Model file for the job. Use its own axes, mm. A direction names the side the tool comes from. Round coordinates to 2 decimals unless told otherwise and drop trailing zeros. Order: outer loops, then holes, each group sorted by start corner. A loop starts at its lowest first (then second) coordinate and runs counter-clockwise, first axis right, second up. Notation, with made-up numbers: (-16, 12.25) - (-3, 12.25) arc R10 ccw to (-3, 30.25) - close; hole circle Ø3 at (-27.5, -6.75). An arc over 180 degrees is marked (long way). Answer as CSV lines item,"result". Start each with the question number.
1. Wall check: line 1 along X through (y, z) = (0.65, -45.5). Give the ranges that are in metal, low to high. Write a range as [from, to].
2. 3-axis set-ups, long thin cutter, end or side, ignore diameter. For faces 4 (the face through (-56, 0.394, -46.454)), 5 (the face through (3, 17, 7.393)), 6 (the face through (-3.9, 7.5, 8.5)), 7 (the face through (5.4, 13, 8)), 8 (the face through (-63.1, 7.9, -45.5)): which of +Z, -Z, +X, -X, +Y, -Y reach the whole face in a straight line?
3. Band-saw the part on D-D on x = -22.5. List the corners of the cut face in (y, z), then the cut area to 3 significant figures.
4. Band-saw the part on A-A on x = 2.7. State how many separate pieces and enclosed holes the cut face has, then the cut area to 3 significant figures.
5. Band-saw the part on B-B on y = 20.5. List the corners of the cut face in (x, z).
6. Band-saw the part on C-C on z = 3.5. List the corners of the cut face in (x, y).
7. Pull direction Z, two halves, no side cores. Call faces 1 (the face through (-3.9, 7.5, -50.4)), 2 (the face through (-63, 3.8, -21)), 3 (the face through (-27, 3, -51)): released by +Z, released by -Z, zero draft, split by the parting line, or undercut.
8. Pin check, flat tips, straight feed: pin 1 Ø1.3 at (x, z) = (-24.5, -50.5) entering from +Y; pin 2 Ø1.6 at (x, z) = (-55.7, 3.5) entering from +Y. Stop position of each tip, or through.
```python
from build123d import *

# Parameters (mm, degrees)
SKETCH1_R            = 0.9999999999999983
SKETCH1_R_2          = 1.0000000000000002
SKETCH1_R_3          = 1.0000000000000013
BOSS_EXTRUDE1_DEPTH  = 0.8
BOSS_EXTRUDE2_DEPTH  = 3
SKETCH3_W            = 2.6000000000000014
SKETCH3_H            = 1.6000000000000156
SKETCH3_W_2          = 5.400000000000002
SKETCH3_H_2          = 1.6066889909461715
SKETCH3_H_3          = 1.6000000000000094
BOSS_EXTRUDE3_DEPTH  = 27
LOFT4_START          = 7.4
LOFT4_DEPTH          = 1.6
LOFT4_START_2        = 7.403174683
LOFT4_2_DEPTH        = 0.596825317
MIRROR6_START        = 7.4
MIRROR6_COPY_1_DEPTH = 1.6
MIRROR6_START_2      = 7.403174683
MIRROR6_COPY_2_DEPTH = 0.596825317
MIRROR6_COPY_3_DEPTH = 1.6
MIRROR6_COPY_4_DEPTH = 0.596825317


with BuildPart() as part:
    # Sketch1 → Boss-Extrude1 (new body)
    with BuildSketch(Plane(origin=(0, 0, 0), x_dir=(1, 0, 0), z_dir=(0, 1, 0))):
        Polygon((0, 0), (5.4, 0), (5.400000000000007, -7.000000000000003), (5.400000000000002, -8.999999999999995), (-58.4, -8.999999999999995), (-61.40000000000001, -8.999999999999995), (-64.4, -8.999999999999995), (-64.4, 51), (-61.40000000000001, 51), (-58.4, 51), (5.400000000000004, 50.99999999999999), (5.400000000000004, 48.99999999999999), (5.4, 42.00000000000001), (0, 41.99999999999999), (-6.07e-15, 48.99999999999999), (-53.00000000000001, 48.99999999999999), (-53.00000000000001, 41.99999999999999), (-58.400000000000006, 41.99999999999999), (-61.40000000000001, 41.99999999999999), (-61.40000000000001, 0), (-58.400000000000006, 0), (-53.00000000000001, -1.73e-15), (-53.00000000000001, -6.999999999999986), (-6.14e-15, -6.999999999999999), align=None)
        with Locations(Location((-55.70000000000001, -3.4999999999999885, 0), (0, 0, 270))):
            Circle(SKETCH1_R, mode=Mode.SUBTRACT)
        with Locations(Location((2.700000000000006, -3.499999999999999, 0), (0, 0, 270))):
            Circle(SKETCH1_R_2, mode=Mode.SUBTRACT)
        with Locations(Location((2.7000000000000015, 45.5, 0), (0, 0, 90))):
            Circle(SKETCH1_R_3, mode=Mode.SUBTRACT)
        with Locations(Location((-55.7, 45.5, 0), (0, 0, 90))):
            Circle(SKETCH1_R, mode=Mode.SUBTRACT)
    extrude(amount=BOSS_EXTRUDE1_DEPTH)

    # Sketch2 → Boss-Extrude2 (add)
    with BuildSketch(Plane(origin=(0, 0.8, 0), x_dir=(1, 0, 0), z_dir=(0, 1, 0))):
        Polygon((-64.4, 51), (5.400000000000002, 51), (5.400000000000002, 49.39999999999999), (-61.800000000000004, 49.39999999999999), (-61.800000000000004, -7.399999999999985), (5.400000000000009, -7.399999999999985), (5.400000000000002, -8.999999999999995), (-64.4, -8.999999999999995), align=None)
    extrude(amount=BOSS_EXTRUDE2_DEPTH)

    # Sketch3 → Boss-Extrude3 (add)
    with BuildSketch(Plane(origin=(0, 3.8, 0), x_dir=(1, 0, 0), z_dir=(0, 1, 0))):
        with Locations((-63.10000000000001, 50.2)):
            Rectangle(SKETCH3_W, SKETCH3_H)
        with Locations((2.700000000000001, 50.2)):
            Rectangle(SKETCH3_W_2, SKETCH3_H)
        with Locations((2.700000000000001, -8.196655504526909)):
            Rectangle(SKETCH3_W_2, SKETCH3_H_2)
        with Locations((-63.10000000000001, -8.19999999999999)):
            Rectangle(SKETCH3_W, SKETCH3_H_3)
    extrude(amount=BOSS_EXTRUDE3_DEPTH)

    # Sketch9 → Loft3 section 0
    with BuildSketch(Plane(origin=(0, 3.8, 0), x_dir=(1, 0, 0), z_dir=(0, 1, 0))):
        with BuildLine():
            Line((-64.4, -7.399999999999985), (-64.4, 0.6000000000000146))
            Line((-64.4, 0.6000000000000146), (-61.800000000000004, 0.6000000000000149))
            Line((-61.800000000000004, 0.6000000000000149), (-61.800000000000004, -7.399999999999985))
            Line((-61.800000000000004, -7.399999999999985), (-64.4, -7.399999999999985))
        make_face()
    # Sketch7 → Loft3 section 1
    with BuildSketch(Plane(origin=(0, 0, 7.399999999999985), x_dir=(-1, 0, -3.903e-14), z_dir=(3.903e-14, 0, -1))):
        with BuildLine():
            Line((64.40000000000235, 3.8), (64.4000000000023, 11.799999999999999))
            Line((64.4000000000023, 11.799999999999999), (61.80000000000229, 11.799999999999997))
            Line((61.80000000000229, 11.799999999999997), (61.80000000000229, 3.8))
            Line((61.80000000000229, 3.8), (64.40000000000235, 3.8))
        make_face()
    loft3 = loft()

    # Loft4: read off the stored shape, not the designer's step
    # Loft4 outline → Loft4 (add)
    with BuildSketch(Plane.XY.offset(LOFT4_START)):
        Polygon((-61.8, 11.8), (-61.8, 3.8), (-53.8, 3.8), align=None)
    loft4 = extrude(amount=LOFT4_DEPTH)

    # Loft4 2 outline → Loft4 2 (add)
    with BuildSketch(Plane(origin=(0, 0, 0), x_dir=(1, 0, 0), z_dir=(0, 0.0008361235760020348, 0.9999996504486218)).offset(LOFT4_START_2)):
        Polygon((-61.8, 11.793814154), (-61.8, 3.793811357), (-53.8, 3.793811357), align=None)
    loft4_2 = extrude(amount=LOFT4_2_DEPTH)

    # Mirror4: Loft3, Loft4, Loft4 2 across plane
    add(loft3.mirror(Plane.XY.offset(-20.999999999999993)))
    add(loft4.mirror(Plane.XY.offset(-20.999999999999993)))
    add(loft4_2.mirror(Plane.XY.offset(-20.999999999999993)))

    # Mirror5: Loft4, Loft4 2 across plane
    add(loft4.mirror(Plane(origin=(-30.700000000000014, 0, 0), x_dir=(0, 0, 1), z_dir=(1, 0, 0))))
    add(loft4_2.mirror(Plane(origin=(-30.700000000000014, 0, 0), x_dir=(0, 0, 1), z_dir=(1, 0, 0))))

    # Mirror6 copy 1 sketch → Mirror6 copy 1 (add)
    with BuildSketch(Plane(origin=(-61.40000000000003, 0, -41.999999999999986), x_dir=(-1, 0, 0), z_dir=(0, 0, -1)).offset(MIRROR6_START)):
        Polygon((-61.8, 11.8), (-61.8, 3.8), (-53.8, 3.8), align=None)
    extrude(amount=MIRROR6_COPY_1_DEPTH)

    # Mirror6 copy 2 sketch → Mirror6 copy 2 (add)
    with BuildSketch(Plane(origin=(-61.40000000000003, 0, -41.999999999999986), x_dir=(-1, 0, 0), z_dir=(0, 0.0008361235760020348, -0.9999996504486218)).offset(MIRROR6_START_2)):
        Polygon((-61.8, 11.793814154), (-61.8, 3.793811357), (-53.8, 3.793811357), align=None)
    extrude(amount=MIRROR6_COPY_2_DEPTH)

    # Mirror6 copy 3 sketch → Mirror6 copy 3 (add)
    with BuildSketch(Plane(origin=(0, 0, -41.999999999999986), x_dir=(1, 0, 0), z_dir=(0, 0, -1)).offset(MIRROR6_START)):
        Polygon((-61.8, -11.8), (-61.8, -3.8), (-53.8, -3.8), align=None)
    extrude(amount=MIRROR6_COPY_3_DEPTH)

    # Mirror6 copy 4 sketch → Mirror6 copy 4 (add)
    with BuildSketch(Plane(origin=(0, 0, -41.999999999999986), x_dir=(1, 0, 0), z_dir=(0, 0.0008361235760020348, -0.9999996504486218)).offset(MIRROR6_START_2)):
        Polygon((-61.8, -11.793814154), (-61.8, -3.793811357), (-53.8, -3.793811357), align=None)
    extrude(amount=MIRROR6_COPY_4_DEPTH)


solid = part.part
```
Reply:
1,line 1,"x = [-64.4, -56.7], [-54.7, -53], [0, 1.7], [3.7, 5.4]"
2,face 4,"+Y, -Y"
2,face 5,"+X, +Y"
2,face 6,"+Z, -Z, +Y"
2,face 7,"+Z, -Z, +X, +Y, -Y"
2,face 8,"+X, -X, +Y"
3,outline,"(0, -51) - (3.8, -51) - (3.8, -49.4) - (0.8, -49.4) - (0.8, -49) - (0, -49) - close; (0, 7) - (0.8, 7) - (0.8, 7.4) - (3.8, 7.4) - (3.8, 9) - (0, 9) - close"
3,area,"12.8 mm2"
4,separate pieces,"4"
4,enclosed holes,"0"
4,area,"107 mm2"
5,outline,"(-64.4, -51) - (-61.8, -51) - (-61.8, -49.4) - (-64.4, -49.4) - close; (-64.4, 7.4) - (-61.8, 7.4) - (-61.8, 9) - (-64.4, 9) - close; (0, -51) - (5.4, -51) - (5.4, -49.4) - (0, -49.4) - close; (0, 7.39) - (5.4, 7.39) - (5.4, 9) - (0, 9) - close"
6,outline,"(-64.4, 0) - (-56.7, 0) - (-56.7, 0.8) - (-61.8, 0.8) - (-61.8, 7.9) - (-64.4, 7.9) - close; (-54.7, 0) - (-53, 0) - (-53, 0.8) - (-54.7, 0.8) - close; (0, 0) - (1.7, 0) - (1.7, 0.8) - (0, 0.8) - close; (3.7, 0) - (5.4, 0) - (5.4, 0.8) - (3.7, 0.8) - close"
7,face 1,"zero draft"
7,face 2,"undercut"
7,face 3,"released by -Z"
8,pin 1,"stops at y = 3.8"
8,pin 2,"passes through"
